Here's how the part is built. I have some questions about the finished solid (model axes, mm). A direction names the side the tool comes from. Round coordinates to 2 decimals unless told otherwise and drop trailing zeros. Write each loop counter-clockwise with the first axis right and the second up, starting at its lowest first coordinate (ties: lowest second). Pieces come first, ordered by that corner, then holes. Notation, with made-up numbers: M -1.5,79.5 L 32.5,79.5 A17 cw 32.5,89.5 Z; hole C -35,-30 d10. An arc over 180 degrees is marked long. Write item = value, one per line. Start each with the question number.
(1) I want a section at D-D (z = -5). List the corners of the cut face in (x, y) for me (3 decimals), and give its area (3 significant figures).
(2) On a 3-axis mill with a long thin cutter (end or side, diameter ignored), from which of +Z, -Z, +X, -X, +Y, -Y can I reach the whole of each face in a straight line? I mean faces 5 (the flat face through (0, 662, 12.385)), 6 (the flat face through (11.88, 661.86, 11.89)), 7 (the flat face through (10.885, 662, 5)). Say none if no direction works.
(3) I want a section at B-B (z = 6.5). List the corners of the cut face in (x, y) for me (3 decimals), and give its area (3 significant figures).
(4) Will these pins go through, and if not, where does the flat tip stop? pin 1 Ø0.8 at (y, z) = (661.5, 3) entering from -X (3 decimals); pin 2 Ø1.1 at (x, y) = (6.5, 662) entering from -Z (3 decimals); pin 3 Ø1 at (y, z) = (662, 17.5) entering from -X; pin 4 Ø0.8 at (x, y) = (-1, 662) entering from +Z (3 decimals).
(5) I want a section at C-C (x = 8). List the corners of the cut face in (y, z) for me (3 decimals), and give its area (3 significant figures).
(6) If we mould it in two halves opening along X, with no side actions, what happens to faces 1 (the flat face through (-11.89, 661.86, -11.88)), 2 (the cylindrical face through (-0.785, 662.896, -0.8)), 3 (the flat face through (0, 662, -12.385)), 4 (the cylindrical face through (-0.8, 662.896, 10.555))? For each: released by +X, released by -X, zero draft, split by the parting line, or undercut.
(7) I want a section at A-A (y = 661.5). List the corners of the cut face in (x, z) for me (3 decimals), and give its area (3 significant figures).
(8) I need wall thicknesses on line 1 along Z through (x, y) = (4, 662.55) (3 decimals); line 2 along Z through (x, y) = (0, 662.65) (3 decimals). Which ranges of each line are inside material? Lowest first, please.
```python
from build123d import *

# Parameters (mm, degrees)
SKETCH008_W     = 24.77
SKETCH008_H     = 24.77
PAD004_DEPTH    = 1.5
SKETCH009_W     = 46.6
SKETCH009_H     = 46.6
PAD005_DEPTH    = 0.6
CHAMFER001_SIZE = 1


with BuildPart() as part:
    # Sketch008 → Pad004 (new body)
    with BuildSketch(Plane.XZ.offset(-662.6)):
        Rectangle(SKETCH008_W, SKETCH008_H)
        with BuildLine():
            Line((-0.115186, -1.115), (10.885, -1.115))
            Line((10.885, -1.115), (10.885, 10.885))
            Line((10.885, 10.885), (-0.115186, 10.885))
            ThreePointArc((-0.115186, 10.885), (-0.822161, 10.592161), (-1.115, 9.885186))
            Line((-1.115, 9.885186), (-1.115, -0.115186))
            ThreePointArc((-1.115, -0.115186), (-0.822161, -0.822161), (-0.115186, -1.115))
        make_face(mode=Mode.SUBTRACT)
    extrude(amount=PAD004_DEPTH)

    # Sketch009 (on Face11 of Pad004) → Pad005 (join)
    with BuildSketch(Plane(origin=(0, 662.6, 0), x_dir=(1, 0, 0), z_dir=(0, 1, 0))):
        Rectangle(SKETCH009_W, SKETCH009_H)
        with BuildLine():
            ThreePointArc((-0.115186, 1.115), (-0.79262, 0.79262), (-1.115, 0.115186))
            Line((-1.115, 0.115186), (-1.115, -9.885186))
            ThreePointArc((-1.115, -9.885186), (-0.79262, -10.56262), (-0.115186, -10.885))
            Line((10.885, -10.885), (-0.115186, -10.885))
            Line((10.885, 1.115), (10.885, -10.885))
            Line((-0.115186, 1.115), (10.885, 1.115))
        make_face(mode=Mode.SUBTRACT)
    extrude(amount=PAD005_DEPTH)

    # Chamfer001
    chamfer001_edges = [part.edges().sort_by_distance(p)[0] for p in [
        (12.385, 661.85, 12.385),
        (-12.385, 661.85, 12.385),
        (-12.385, 661.85, -12.385),
        (12.385, 661.85, -12.385),
        (23.3, 662.9, 23.3),
        (-23.3, 662.9, 23.3),
        (23.3, 662.9, -23.3),
        (-23.3, 662.9, -23.3),
    ]]
    chamfer(chamfer001_edges, length=CHAMFER001_SIZE)


solid = part.part
```
Returned:
q1.outline = M -23.3,662.6 L -12.385,662.6 L -12.385,661.1 L 12.385,661.1 L 12.385,662.6 L 23.3,662.6 L 23.3,663.2 L -23.3,663.2 Z
q1.area = 65.1 mm²
q2.face_5 = +Z, +X, -X, -Y
q2.face_6 = +Z, +X, -Y
q2.face_7 = +Y, -Y
q3.outline = M -23.3,662.6 L -12.385,662.6 L -12.385,661.1 L -1.115,661.1 L -1.115,663.2 L -23.3,663.2 Z; M 10.885,661.1 L 12.385,661.1 L 12.385,662.6 L 23.3,662.6 L 23.3,663.2 L 10.885,663.2 Z
q3.area = 39.9 mm²
q4.pin_1 = -12.385
q4.pin_2 = -12.385
q4.pin_3 = through
q4.pin_4 = 12.385
q5.outline = M 661.1,-12.385 L 662.6,-12.385 L 662.6,-23.3 L 663.2,-23.3 L 663.2,-1.115 L 661.1,-1.115 Z; M 661.1,10.885 L 663.2,10.885 L 663.2,23.3 L 662.6,23.3 L 662.6,12.385 L 661.1,12.385 Z
q5.area = 39.9 mm²
q6.face_1 = released by -X
q6.face_2 = undercut
q6.face_3 = zero draft
q6.face_4 = undercut
q7.outline = M -12.385,-11.385 L -11.385,-12.385 L 11.385,-12.385 L 12.385,-11.385 L 12.385,11.385 L 11.385,12.385 L -11.385,12.385 L -12.385,11.385 Z; hole M -1.115,-0.115 A1 ccw -0.115,-1.115 L 10.885,-1.115 L 10.885,10.885 L -0.115,10.885 A1 ccw -1.115,9.885 Z
q7.area = 468 mm²
q8.line_1 = -12.385 to -1.115, 10.885 to 12.385
q8.line_2 = -23.3 to -1.115, 10.885 to 23.3
